Verification items for this drawing (mm, ordinates from the low corner). Round coordinates to 2 decimals unless told otherwise and drop trailing zeros. Order: outer loops, then holes, each group sorted by start corner. A loop starts at its lowest first (then second) coordinate and runs counter-clockwise, first axis right, second up.
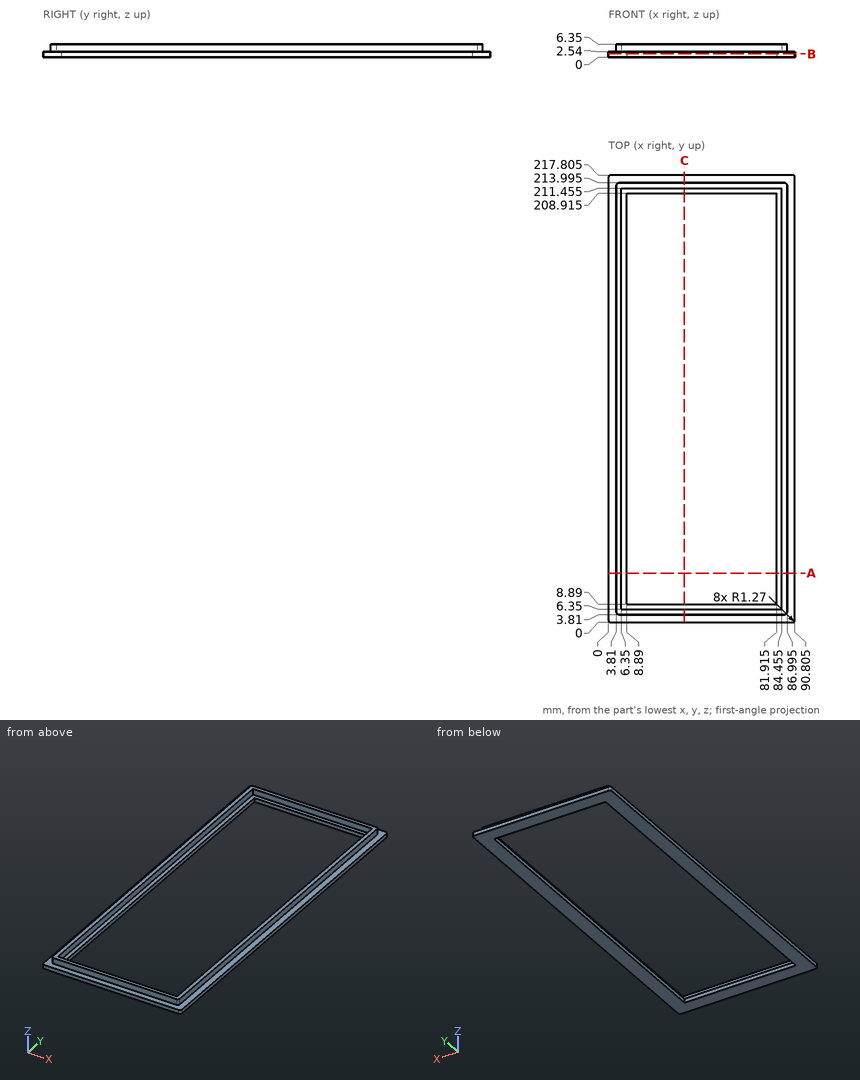
Item 1: Scan lines: line 1 along X through (y, z) = (186.5, 3.25) (3 decimals); line 2 along Y through (x, z) = (22.5, 5.5) (3 decimals); line 3 along X through (y, z) = (194, 1.25) (3 decimals). Record each from-to range of solid material in increasing order.
Answer:
line 1: x = 3.81 to 6.35, 84.455 to 86.995
line 2: y = 3.81 to 6.35, 211.455 to 213.995
line 3: x = 0 to 8.89, 81.915 to 90.805
Item 2: Sectioned sample at C-C (x = 37). Record the cut outline in (y, z) (3 decimals), and give its area (3 significant figures).
Answer:
outline: (0, 0) - (8.89, 0) - (8.89, 2.54) - (6.35, 2.54) - (6.35, 6.35) - (3.81, 6.35) - (3.81, 2.54) - (0, 2.54) - close; (208.915, 0) - (217.805, 0) - (217.805, 2.54) - (213.995, 2.54) - (213.995, 6.35) - (211.455, 6.35) - (211.455, 2.54) - (208.915, 2.54) - close
area: 64.5 mm2
Item 3: Sectioned sample at B-B (z = 1.5). Record the cut outline in (x, y) (3 decimals).
Answer:
outline: (0, 1.27) arc R1.27 ccw to (1.27, 0) - (89.535, 0) arc R1.27 ccw to (90.805, 1.27) - (90.805, 216.535) arc R1.27 ccw to (89.535, 217.805) - (1.27, 217.805) arc R1.27 ccw to (0, 216.535) - close; hole (8.89, 8.89) - (81.915, 8.89) - (81.915, 208.915) - (8.89, 208.915) - close
Item 4: Sectioned sample at A-A (y = 24). Record the cut outline in (x, z) (3 decimals).
Answer:
outline: (0, 0) - (8.89, 0) - (8.89, 2.54) - (6.35, 2.54) - (6.35, 6.35) - (3.81, 6.35) - (3.81, 2.54) - (0, 2.54) - close; (81.915, 0) - (90.805, 0) - (90.805, 2.54) - (86.995, 2.54) - (86.995, 6.35) - (84.455, 6.35) - (84.455, 2.54) - (81.915, 2.54) - close
Item 5: Go/stop test with flat-tipped pins: P1, Ø3, axis at y = 71, z = 4.5, coming from the -X side; P2, Ø1.9, axis at x = 43.5, z = 4, coming from the -Y side; P3, Ø1.1, axis at x = 54, z = 3.5, coming from the +Y side (3 decimals). Record where each tip stops, or that it passes through.
Answer:
P1: stops at x = 3.81
P2: stops at y = 3.81
P3: stops at y = 213.995
